from build123d import *

# Parameters (mm, degrees)
EXTRUDE001_DEPTH                     = 100
EXTRUDE001_ONTO_SKETCH001_ROLL_ANGLE = 90
FILLET003_R                          = 80
FILLET003_PLACEMENT_ANGLE            = 90
EXTRUDE_DEPTH                        = 400
CHAMFER_SIZE                         = 40
FILLET_R                             = 5
FILLET001_R                          = 5
FILLET002_R                          = 5
FUSION001_PLACEMENT_ANGLE            = -90


with BuildPart() as pas001:
    # Sketch001 as drawn → Extrude001 (new)
    with BuildSketch(Plane.XY):
        Polygon((-750, 325), (-620, -225), (620, -225), (850, 325), align=None)
    extrude(amount=-EXTRUDE001_DEPTH)


with BuildPart() as pas001_1:
    # Extrude001 onto Sketch001 roll: moved
    add(pas001.part.rotate(Axis((0, 0, 0), (1, 0, 0)), EXTRUDE001_ONTO_SKETCH001_ROLL_ANGLE))


with BuildPart() as pas001_2:
    # Extrude001 onto Sketch001 placement: moved
    add(pas001_1.part)

    # Fillet003
    fillet003_edges = [pas001_2.edges().sort_by_distance(p)[0] for p in [
        (-750, 50, 325),
        (-620, 50, -225),
        (620, 50, -225),
        (850, 50, 325),
    ]]
    fillet(fillet003_edges, radius=FILLET003_R)


with BuildPart() as pas001_3:
    # Fillet003 placement: moved
    add(pas001_2.part.moved(Location((-380, 0, 0))).rotate(Axis((-380, 0, 0), (0, 0, 1)), FILLET003_PLACEMENT_ANGLE))


with BuildPart() as fusion:
    # Sketch → Extrude (new body)
    with BuildSketch(Plane.XY):
        Polygon((-380, 600), (-380, -80), (-300, -200), (-300, -600), (300, -600), (300, -200), (380, -80), (380, 600), align=None)
    extrude(amount=EXTRUDE_DEPTH)

    # Chamfer
    chamfer_edges = [fusion.edges().sort_by_distance(p)[0] for p in [
        (0, -600, 0),
        (0, -600, 400),
        (0, 600, 0),
        (0, 600, 400),
    ]]
    chamfer(chamfer_edges, length=CHAMFER_SIZE)

    # Fillet
    fillet_edges = [fusion.edges().sort_by_distance(p)[0] for p in [
        (-380, 600, 200),
        (-380, 240, 0),
        (-380, 240, 400),
        (-340, -140, 0),
        (-300, -380, 0),
        (-340, -140, 400),
        (-300, -380, 400),
        (-300, -600, 200),
        (-300, -580, 20),
        (-300, -580, 380),
    ]]
    fillet(fillet_edges, radius=FILLET_R)

    # Fillet001
    fillet001_edges = [fusion.edges().sort_by_distance(p)[0] for p in [
        (-380, 580, 20),
        (-380, 580, 380),
    ]]
    fillet(fillet001_edges, radius=FILLET001_R)

    # Fillet002
    fillet002_edges = [fusion.edges().sort_by_distance(p)[0] for p in [
        (380, 600, 200),
        (380, 580, 20),
        (380, 580, 380),
        (380, 238.964466, 0),
        (340, -140, 0),
        (300, -380, 0),
        (380, 238.964466, 400),
        (340, -140, 400),
        (300, -380, 400),
        (300, -580, 20),
        (300, -600, 200),
        (300, -580, 380),
    ]]
    fillet(fillet002_edges, radius=FILLET002_R)

    # Fusion: union Pas001
    add(pas001_3.part)


with BuildPart() as obj1:
    # Part__Mirroring: instance of Pas001
    add(pas001_3.part.mirror(Plane(origin=(0, 0, 0), x_dir=(0, -1, 0), z_dir=(1, 0, 0))))

    # Fusion001: union Fusion
    add(fusion.part)


with BuildPart() as obj1_1:
    # Fusion001 placement: moved
    add(obj1.part.rotate(Axis((0, 0, 0), (0, 0, 1)), FUSION001_PLACEMENT_ANGLE))


solid = obj1_1.part
Check sheet for the modelled part. Datum: model origin and axes. Units: mm. A direction names the side the tool comes from. Round coordinates to 2 decimals unless told otherwise and drop trailing zeros. Loops run counter-clockwise (first coordinate to the right, second up) from the corner with the lowest first, then second, coordinate; pieces in that order, holes last. Notation, with made-up numbers: (48, 6) - (66, 6) arc R18 cw to (66, 30) - close; hole circle Ø11 at (69.25, 9). An arc over 180 degrees is marked (long way). Answer as CSV lines item,"result". Start each with the question number.
Item 1: Section check A-A (z = -122.5). Record the boundary of the cut face in (x, y).
Item 2: Section check C-C (x = 303.5). Record the boundary of the cut face in (y, z).
Item 3: Section check B-B (y = -230). Record the boundary of the cut face in (x, z), and give its area (3 significant figures).
Item 4: Section check D-D (z = 160.5). Record the boundary of the cut face in (x, y).
Item 5: Release check for a two-part mould opening along X. For faces 1 (the cylindrical face through (-140.645, 337.763, 398.574)), 2 (the cylindrical face through (578.73, 378.57, 20.85)), 3 (the cylindrical face through (578.73, 378.57, 379.15)), 4 (the flat face through (50, 429, 325)) record: +X half, -X half, draft (parallel to the pull), parting line (faces both ways), or undercut.
Item 6: Scan lines: line 1 (Y direction, x = -289, z = 300); line 2 (Y direction, x = -613, z = 65); line 3 (Y direction, x = -144, z = 118.5). Record each from-to range of solid material in increasing order. Write a range as [from, to].
Item 7: Set-up check for faces 5 (the flat face through (-580, 4, 20)), 6 (the flat face through (-395, 300, 197)), 7 (the flat face through (600, -5, 198)), 8 (the flat face through (-3, -429, -225)), 9 (the cylindrical face through (-578.66, -298.57, 379.22)): record each of +Z, -Z, +X, -X, +Y, -Y from which the full face is reachable in a straight line by a thin tool's end or side.
Item 8: Depth check by flat-ended pin: P1, Ø3, axis at x = -499.5, y = -142.5, coming from the -Z side; P2, Ø1.5, axis at y = 339, z = 308, coming from the +X side; P3, Ø5, axis at y = 101, z = 211, coming from the -X side. Enter the tip coordinate at first touch or a pass-through.
Report:
1,outline,"(-644.23, -480) - (662.86, -480) - (662.86, -380) - (-644.23, -380) - close; (-644.23, 380) - (662.86, 380) - (662.86, 480) - (-644.23, 480) - close"
2,outline,"(-480, -225) - (-380, -225) - (-380, 5) arc R5 ccw to (-375, 0) - (375, 0) arc R5 ccw to (380, 5) - (380, -225) - (480, -225) - (480, 325) - (380, 325) - (380, 395) arc R5 ccw to (375, 400) - (-375, 400) arc R5 ccw to (-380, 395) - (-380, 325) - (-480, 325) - close"
3,outline,"(-600, 40) - (-560, 0) - (557.93, 0) arc R5 ccw to (561.46, 1.46) - (598.54, 38.54) arc R5 ccw to (600, 42.07) - (600, 357.93) arc R5 ccw to (598.54, 361.46) - (561.46, 398.54) arc R5 ccw to (557.93, 400) - (-560, 400) - (-600, 360) - close"
3,area,"477,000 mm2"
4,outline,"(-711.12, -480) - (781.21, -480) - (781.21, -380) - (595, -380) arc R5 ccw to (600, -375) - (600, 375) arc R5 ccw to (595, 380) - (781.21, 380) - (781.21, 480) - (-711.12, 480) - (-711.12, 380) - (-80, 380) - (-200, 300) - (-595, 300) arc R5 ccw to (-600, 295) - (-600, -295) arc R5 ccw to (-595, -300) - (-200, -300) - (-80, -380) - (-711.12, -380) - close"
5,face 1,"-X half"
5,face 2,"undercut"
5,face 3,"+X half"
5,face 4,"draft"
6,line 1,"y = [-480, -380], [-300, 300], [380, 480]"
6,line 2,"y = [-480, -380], [380, 480]"
6,line 3,"y = [-480, -380], [-337.33, 337.33], [380, 480]"
7,face 5,"-Z, -X"
7,face 6,"+Z, -Z, -X"
7,face 7,"+Z, -Z, +X"
7,face 8,"-Z, +X, -X, +Y, -Y"
7,face 9,"+Z, -X, -Y"
8,P1,"stops at z = 0"
8,P2,"stops at x = 600"
8,P3,"stops at x = -600"
